Build history of the part. All positions in model axes, mm. Face numbers are marked on the shaded views. A direction names the side the tool comes from. Coordinates: 2 decimals unless noted, no trailing zeros. Write each loop counter-clockwise with the first axis right and the second up, starting at its lowest first coordinate (ties: lowest second). Pieces come first, ordered by that corner, then holes. Notation, with made-up numbers: M 3.25,47.5 L 20.25,47.5 A33 ccw 20.25,77.5 Z; hole C 9.25,-22 d9. An arc over 180 degrees is marked long. Use CSV: the item, a comma, the result in double quotes. Start each with the question number.
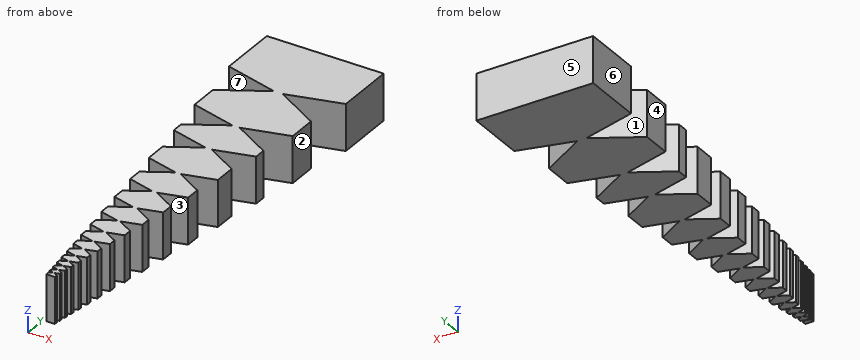
```python
from build123d import *

# Parameters (mm, degrees)
BOSS_EXTRUDE1_DEPTH = 10


with BuildPart() as part:
    # spiral_flat → Boss-Extrude1 (new body)
    with BuildSketch(Plane.XY):
        with BuildLine():
            Line((0, 93.978977978), (-12.645458185, 93.978977978))
            Line((-12.645458185, 93.978977978), (-12.645458185, 81.037355698))
            Line((-12.645458185, 81.037355698), (-0.948409364, 77.903140912))
            Line((-0.948409364, 77.903140912), (-10.613540319, 72.322974954))
            Line((-10.613540319, 72.322974954), (-10.613540319, 66.071506497))
            Line((-10.613540319, 66.071506497), (-0.785032027, 63.437965637))
            Line((-0.785032027, 63.437965637), (-8.90811835, 58.748099562))
            Line((-8.90811835, 58.748099562), (-8.90811835, 56.263194352))
            Line((-8.90811835, 56.263194352), (-0.679092373, 54.058233487))
            Line((-0.679092373, 54.058233487), (-7.476729738, 50.133615724))
            Line((-7.476729738, 50.133615724), (-7.476729738, 45.433932588))
            Line((-7.476729738, 45.433932588), (-0.56075473, 43.58080267))
            Line((-0.56075473, 43.58080267), (-6.275341816, 40.281484278))
            Line((-6.275341816, 40.281484278), (-6.275341816, 37.158488644))
            Line((-6.275341816, 37.158488644), (-0.470650636, 35.603126331))
            Line((-0.470650636, 35.603126331), (-5.266997241, 32.833954327))
            Line((-5.266997241, 32.833954327), (-5.266997241, 30.212772905))
            Line((-5.266997241, 30.212772905), (-0.395024793, 28.907331822))
            Line((-0.395024793, 28.907331822), (-4.420677113, 26.583120371))
            Line((-4.420677113, 26.583120371), (-4.420677113, 24.383079269))
            Line((-4.420677113, 24.383079269), (-0.331702205, 23.287441744))
            Line((-0.331702205, 23.287441744), (-3.710346757, 21.336780402))
            Line((-3.710346757, 21.336780402), (-3.710346757, 19.490083441))
            Line((-3.710346757, 19.490083441), (-0.278697859, 18.57057589))
            Line((-0.278697859, 18.57057589), (-3.114154847, 16.933524034))
            Line((-3.114154847, 16.933524034), (-3.114154847, 15.383475192))
            Line((-3.114154847, 15.383475192), (-0.233600822, 14.611633067))
            Line((-0.233600822, 14.611633067), (-2.613761206, 13.237446829))
            Line((-2.613761206, 13.237446829), (-2.613761206, 11.936656031))
            Line((-2.613761206, 11.936656031), (-0.19603209, 11.288827467))
            Line((-0.19603209, 11.288827467), (-2.19377262, 10.135431435))
            Line((-2.19377262, 10.135431435), (-2.19377262, 9.043614273))
            Line((-2.19377262, 9.043614273), (-0.164761066, 8.499942265))
            Line((-0.164761066, 8.499942265), (-1.841269317, 7.532009775))
            Line((-1.841269317, 7.532009775), (-1.841269317, 6.615509703))
            Line((-1.841269317, 6.615509703), (-0.138243102, 6.159185204))
            Line((-0.138243102, 6.159185204), (-1.545407517, 5.346758451))
            Line((-1.545407517, 5.346758451), (-1.545407517, 4.577583331))
            Line((-1.545407517, 4.577583331), (-0.115905564, 4.194549437))
            Line((-0.115905564, 4.194549437), (-1.297085859, 3.512594676))
            Line((-1.297085859, 3.512594676), (-1.297085859, 2.867070252))
            Line((-1.297085859, 2.867070252), (-0.097336711, 2.545598437))
            Line((-0.097336711, 2.545598437), (-1.088665421, 1.973254539))
            Line((-1.088665421, 1.973254539), (-1.088665421, 1.431435829))
            Line((-1.088665421, 1.431435829), (-0.081649907, 1.161606835))
            Line((-0.081649907, 1.161606835), (-0.913734731, 0.681202438))
            Line((-0.913734731, 0.681202438), (-0.913734731, 0))
            Line((-0.913734731, 0), (0, 0))
            add(Edge.make_bspline(
                [(0, 0), (0, 0.387202278), (0, 1.235735091), (0, 2.633918237), (0, 4.299777693), (0, 6.284558969), (0, 8.649318312), (0, 11.466800933), (0, 14.823678808), (0, 18.8232169), (0, 23.588449819), (0, 29.265966632), (0, 36.030420274), (0, 44.414054162), (0, 53.692333931), (0, 65.133113345), (0, 78.440028176), (0, 88.620365623), (0, 93.978977978)],
                knots=[0, 0, 0, 0, 0.012360284, 0.027086892, 0.044632848, 0.065537904, 0.090445145, 0.120120773, 0.155477676, 0.19760351, 0.247794158, 0.307593596, 0.378841387, 0.463729268, 0.575216231, 0.675022936, 0.828942202, 1, 1, 1, 1], degree=3))
        make_face()
        with BuildLine():
            Line((12.645458185, 93.978977978), (0, 93.978977978))
            add(Edge.make_bspline(
                [(0, 0), (0, 0.387202278), (0, 1.235735091), (0, 2.633918237), (0, 4.299777693), (0, 6.284558969), (0, 8.649318312), (0, 11.466800933), (0, 14.823678808), (0, 18.8232169), (0, 23.588449819), (0, 29.265966632), (0, 36.030420274), (0, 44.414054162), (0, 53.692333931), (0, 65.133113345), (0, 78.440028176), (0, 88.620365623), (0, 93.978977978)],
                knots=[0, 0, 0, 0, 0.012360284, 0.027086892, 0.044632848, 0.065537904, 0.090445145, 0.120120773, 0.155477676, 0.19760351, 0.247794158, 0.307593596, 0.378841387, 0.463729268, 0.575216231, 0.675022936, 0.828942202, 1, 1, 1, 1], degree=3))
            Line((0, 0), (0.913734731, 0))
            Line((0.913734731, 0), (0.913734731, 0.681202438))
            Line((0.913734731, 0.681202438), (0.081649907, 1.161606835))
            Line((0.081649907, 1.161606835), (1.088665421, 1.431435829))
            Line((1.088665421, 1.431435829), (1.088665421, 1.973254539))
            Line((1.088665421, 1.973254539), (0.097336711, 2.545598437))
            Line((0.097336711, 2.545598437), (1.297085859, 2.867070252))
            Line((1.297085859, 2.867070252), (1.297085859, 3.512594676))
            Line((1.297085859, 3.512594676), (0.115905564, 4.194549437))
            Line((0.115905564, 4.194549437), (1.545407517, 4.577583331))
            Line((1.545407517, 4.577583331), (1.545407517, 5.346758451))
            Line((1.545407517, 5.346758451), (0.138243102, 6.159185204))
            Line((0.138243102, 6.159185204), (1.841269317, 6.615509703))
            Line((1.841269317, 6.615509703), (1.841269317, 7.532009775))
            Line((1.841269317, 7.532009775), (0.164761066, 8.499942265))
            Line((0.164761066, 8.499942265), (2.19377262, 9.043614273))
            Line((2.19377262, 9.043614273), (2.19377262, 10.135431435))
            Line((2.19377262, 10.135431435), (0.19603209, 11.288827467))
            Line((0.19603209, 11.288827467), (2.613761206, 11.936656031))
            Line((2.613761206, 11.936656031), (2.613761206, 13.237446829))
            Line((2.613761206, 13.237446829), (0.233600822, 14.611633067))
            Line((0.233600822, 14.611633067), (3.114154847, 15.383475192))
            Line((3.114154847, 15.383475192), (3.114154847, 16.933524034))
            Line((3.114154847, 16.933524034), (0.278697859, 18.57057589))
            Line((0.278697859, 18.57057589), (3.710346757, 19.490083441))
            Line((3.710346757, 19.490083441), (3.710346757, 21.336780402))
            Line((3.710346757, 21.336780402), (0.331702205, 23.287441744))
            Line((0.331702205, 23.287441744), (4.420677113, 24.383079269))
            Line((4.420677113, 24.383079269), (4.420677113, 26.583120371))
            Line((4.420677113, 26.583120371), (0.395024793, 28.907331822))
            Line((0.395024793, 28.907331822), (5.266997241, 30.212772905))
            Line((5.266997241, 30.212772905), (5.266997241, 32.833954327))
            Line((5.266997241, 32.833954327), (0.470650636, 35.603126331))
            Line((0.470650636, 35.603126331), (6.275341816, 37.158488644))
            Line((6.275341816, 37.158488644), (6.275341816, 40.281484278))
            Line((6.275341816, 40.281484278), (0.56075473, 43.58080267))
            Line((0.56075473, 43.58080267), (7.476729738, 45.433932588))
            Line((7.476729738, 45.433932588), (7.476729738, 50.133615724))
            Line((7.476729738, 50.133615724), (0.679092373, 54.058233487))
            Line((0.679092373, 54.058233487), (8.90811835, 56.263194352))
            Line((8.90811835, 56.263194352), (8.90811835, 58.748099562))
            Line((8.90811835, 58.748099562), (0.785032027, 63.437965637))
            Line((0.785032027, 63.437965637), (10.613540319, 66.071506497))
            Line((10.613540319, 66.071506497), (10.613540319, 72.322974954))
            Line((10.613540319, 72.322974954), (0.948409364, 77.903140912))
            Line((0.948409364, 77.903140912), (12.645458185, 81.037355698))
            Line((12.645458185, 81.037355698), (12.645458185, 93.978977978))
        make_face()
    extrude(amount=BOSS_EXTRUDE1_DEPTH)


solid = part.part
```
1. Slice it at A-A (y = 39). List the corners of the cut face in (x, z), and give its area (3 significant figures).
2. Slice it at B-B (y = 69). List the corners of the cut face in (x, z), and give its area (3 significant figures).
3. 3-axis set-ups, long thin cutter, end or side, ignore diameter. For the marked faces 1, 2, 3 and 4: which of +Z, -Z, +X, -X, +Y, -Y reach the whole face in a straight line?
4. Drill centre lines: line 1 along Y through (x, z) = (4.5, 1.75); line 2 along X through (y, z) = (63, 4); line 3 along X through (y, z) = (58.5, 6). Where is each one in solid material? Low to high. Write a range as from..to.
5. Flat gauge pins, fed straight in: pin 1 (1 mm diameter, centred on y = 7, z = 7, fed in from +X); pin 2 (2 mm diameter, centred on x = -8.5, y = 50.5, fed in from +Z); pin 3 (1.5 mm diameter, centred on y = 20.5, z = 7, fed in from +X); pin 4 (1 mm diameter, centred on y = 12.5, z = 6, fed in from -X). Where does each tip first touch, or does it go through?
6. Pull direction Y, two halves, no side cores. Call the marked faces 5, 6 and 7: pulls with the +Y half, pulls with the -Y half, needs draft (parallel to the pull), parting line crosses it, or undercut.
Established:
1,outline,"M -6.28,0 L 6.28,0 L 6.28,10 L -6.28,10 Z"
1,area,"126 mm2"
2,outline,"M -10.61,0 L 10.61,0 L 10.61,10 L -10.61,10 Z"
2,area,"212 mm2"
3,face 1,"+Z, -Z, -X"
3,face 2,"+Z, -Z, +X, -Y"
3,face 3,"+Z, -Z, +X"
3,face 4,"+Z, -Z, -X, -Y"
4,line 1,"y = 30.01..33.28, 36.68..41.31, 44.64..51.85, 55.08..61.29, 64.43..75.85, 78.85..93.98"
4,line 2,"x = -1.54..1.54"
4,line 3,"x = -8.91..8.91"
5,pin 1,"stops at x = 1.84"
5,pin 2,"passes through"
5,pin 3,"stops at x = 3.71"
5,pin 4,"stops at x = -2.61"
6,face 5,"pulls with the +Y half"
6,face 6,"needs draft"
6,face 7,"undercut"
